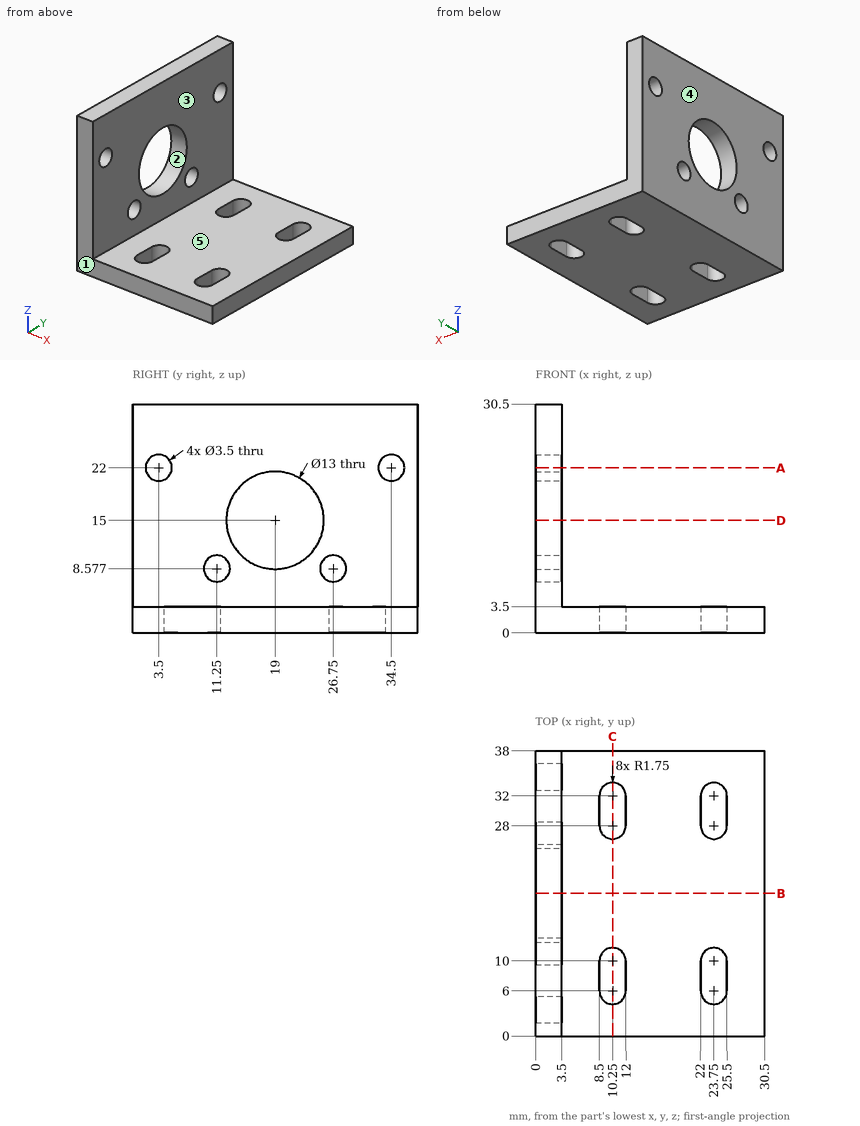
Design review of the part shown in the three views and the two pictorial views. Dimensions are in mm from the part's minimum x, y and z. A direction names the side the tool comes from. Coordinates: 2 decimals unless noted, no trailing zeros. Loops run counter-clockwise (first coordinate to the right, second up) from the corner with the lowest first, then second, coordinate; pieces in that order, holes last.
(1) Consider section D-D, the plane z = 15. Give the boundary of the cut face in (x, y).
Determined:
outline: (0, 0) - (3.5, 0) - (3.5, 12.5) - (0, 12.5) - close; (0, 25.5) - (3.5, 25.5) - (3.5, 38) - (0, 38) - close
(2) Draft analysis for pull direction Y (two halves, no side actions). For the marked faces 1, 2 and 3, state which applies: +Y half, -Y half, draft (parallel to the pull), parting line (faces both ways), or undercut.
Determined:
face 1: -Y half
face 2: undercut
face 3: draft
(3) Tool access review of the marked faces 4 and 5: name each direction out of +Z, -Z, +X, -X, +Y, -Y from which nothing blocks a thin tool from reaching the whole face with its end or side.
Determined:
face 4: +Z, -Z, -X, +Y, -Y
face 5: +Z, +X, +Y, -Y
(4) Consider section A-A, the plane z = 22. Give the boundary of the cut face in (x, y).
Determined:
outline: (0, 0) - (3.5, 0) - (3.5, 1.75) - (0, 1.75) - close; (0, 5.25) - (3.5, 5.25) - (3.5, 32.75) - (0, 32.75) - close; (0, 36.25) - (3.5, 36.25) - (3.5, 38) - (0, 38) - close
(5) Consider section B-B, the plane y = 19. Give the boundary of the cut face in (x, z).
Determined:
outline: (0, 0) - (30.5, 0) - (30.5, 3.5) - (3.5, 3.5) - (3.5, 8.5) - (0, 8.5) - close; (0, 21.5) - (3.5, 21.5) - (3.5, 30.5) - (0, 30.5) - close
(6) Consider section C-C, the plane x = 10.25. Give the boundary of the cut face in (y, z).
Determined:
outline: (0, 0) - (4.25, 0) - (4.25, 3.5) - (0, 3.5) - close; (11.75, 0) - (26.25, 0) - (26.25, 3.5) - (11.75, 3.5) - close; (33.75, 0) - (38, 0) - (38, 3.5) - (33.75, 3.5) - close
(7) Wall thickness on L1, parallel to Z at x = 14.5, y = 34.5; L2, parallel to Z at x = 1.55, y = 11.25: over which ranges is each line inside the solid? List them lowest first.
Determined:
L1: z = 0 to 3.5
L2: z = 0 to 6.83, 10.33 to 30.5
(8) Insertion check: P1, Ø15, axis at y = 19, z = 15, coming from the -X side; P2, Ø13.5, axis at x = 17, y = 22.5, coming from the +Z side; P3, Ø8, axis at y = 15, z = 23, coming from the +X side. Each pin has a flat end and moves straight along its axis. Give the tip position at first contact, or say it passes through.
Determined:
P1: stops at x = 0
P2: stops at z = 3.5
P3: stops at x = 3.5
